Here's how the part is built. I have some questions about the finished solid (model axes, mm). A direction names the side the tool comes from. Give positions to 0.01 mm unless a question says otherwise; leave off trailing zeros. Loops run counter-clockwise (first coordinate to the right, second up) from the corner with the lowest first, then second, coordinate; pieces in that order, holes last. Notation, with made-up numbers: (-38.5, 71.5) - (18.5, 71.5) arc R16 cw to (18.5, 95.5) - close; hole circle Ø8 at (42, 88.25). An arc over 180 degrees is marked (long way). Use one line per item in the form item = value.
Autodesk Inventor part; units mm, degrees
ref_plane "YZ Plane" through (0, 0, 0) normal (1, 0, 0) x (0, 1, 0)
ref_plane "XZ Plane" through (0, 0, 0) normal (0, 1, 0) x (-1, 0, 0)
ref_plane "XY Plane" through (0, 0, 0) normal (0, 0, 1) x (1, 0, 0)
sketch "Sketch1" plane through (0, 0, 0) normal (0, 1, 0) x (-1, 0, 0)
  line L0 (27.5, 37.5) -> (-27.5, 37.5)
  line L1 (-27.5, 37.5) -> (-27.5, -37.5)
  line L2 (-27.5, -37.5) -> (27.5, -37.5)
  line L3 (27.5, -37.5) -> (27.5, 37.5)
  line L4 (27.5, 37.5) -> (-27.5, -37.5) construction
  line L5 (-27.5, 37.5) -> (27.5, -37.5) construction
  point P0 (0, 0)
  dimension "d0" = 75
  dimension "d1" = 55
extrude "Extrusion1" add sketch "Sketch1" along normal blind 18
sketch "Sketch2" plane through (0, 18, 0) normal (0, 1, 0) x (1, 0, 0)
  line L0 (-27.5, -37.5) -> (27.5, -37.5)
  line L1 (-8.5, -37.5) -> (-8.5, 37.5)
  line L2 (27.5, -37.5) -> (27.5, 37.5)
  line L3 (-8.5, 37.5) -> (27.5, 37.5)
  line L4 (-8.5, -37.5) -> (27.5, -37.5)
  dimension "d4" = 36
extrude "Extrusion2" add sketch "Sketch2" along normal blind 7
sketch "Sketch3" plane through (0, 18, 0) normal (0, 1, 0) x (1, 0, 0)
  line L0 (27.5, 37.5) -> (-27.5, 37.5)
  line L1 (-27.5, 37.5) -> (-27.5, -37.5)
  line L2 (-8.5, 37.5) -> (-8.5, -37.5)
  circle A0 centre (-18, 25.4407) radius 5.5
  circle A1 centre (-18, -24.214) radius 5.5
  point P0 (0, 0)
  dimension "d9" = 19
  dimension "d10" = 11
  dimension "d11" = 11
extrude "Extrusion3" cut sketch "Sketch3" against normal blind 7
sketch "Sketch4" plane through (-18, 11, -25.4407) normal (0, 1, 0) x (1, 0, 0)
  circle A0 centre (0, 0) radius 3.2
  circle A1 centre (0, -49.6547) radius 5.5
  circle A2 centre (0, -49.6547) radius 3.2
  point P0 (18, -25.4407)
  dimension "d14" = 6.4
  dimension "d15" = 6.4
extrude "Extrusion4" cut sketch "Sketch4" against normal blind 15 contours A0 | A2
sketch "Sketch5" plane through (0, 25, 0) normal (0, 1, 0) x (1, 0, 0)
  circle A0 centre (19.5, 0) radius 7.5
  circle A1 centre (4.5, 10.5) radius 7.5
  circle A2 centre (4.5, -10.5) radius 7.5
  line L0 (27.5, -37.5) -> (27.5, 37.5)
  point P0 (0, 0)
  dimension "d18" = 15
  dimension "d19" = 15
  dimension "d20" = 15
  dimension "d21" = 23
  dimension "d22" = 23
  dimension "d23" = 8
  dimension "d26" = 21
  dimension "d27" = 10.5
  dimension "d28" = 10.5
extrude "Extrusion5" cut sketch "Sketch5" against normal blind 10
sketch "Sketch6" plane through (4.5, 15, 10.5) normal (0, 1, 0) x (1, 0, 0)
  circle A0 centre (0, 0) radius 4.2
  circle A1 centre (0, 21) radius 7.5
  circle A2 centre (0, 21) radius 4.2
  circle A3 centre (15, 10.5) radius 7.5
  circle A4 centre (15, 10.5) radius 4.2
  point P0 (-4.5, 10.5)
  dimension "d29" = 8.4
  dimension "d30" = 8.4
  dimension "d31" = 8.4
extrude "Extrusion6" cut sketch "Sketch6" against normal blind 20 contours A0 | A2 | A4
properties part number "Feste Backe"
(1) For P1, Ø9, axis at x = -16, z = -24, coming from the +Y side; P2, Ø9.5, axis at x = 4.5, z = -10.5, coming from the +Y side; P3, Ø4, axis at x = -18, z = 24.214, coming from the +Y side; P4, Ø6.5, axis at x = -18, z = 24.214, coming from the +Y side, each with a flat end and sliding along its axis, tell me the tip position at first contact or that it passes through.
Geometry says:
P1 = 18
P2 = 15
P3 = through
P4 = 11
(2) If we section it at D-D (x = 20.5): List the corners of the cut face in (y, z) for me, plus the area to 3 significant figures.
Geometry says:
outline = (0, -37.5) - (25, -37.5) - (25, -7.43) - (15, -7.43) - (15, -4.08) - (0, -4.08) - close; (0, 4.08) - (15, 4.08) - (15, 7.43) - (25, 7.43) - (25, 37.5) - (0, 37.5) - close
area = 1,600 mm²
(3) If I drill on probe 1 along Z at (x, y) = (-18, 5.25); probe 2 along Z at (x, y) = (4.5, 8); probe 3 along X at (y, z) = (23.5, 0), over which ranges is the centre line in solid material (lowest first)?
Geometry says:
probe_1 = -37.5 to -28.64, -22.24 to 21.01, 27.41 to 37.5
probe_2 = -37.5 to -14.7, -6.3 to 6.3, 14.7 to 37.5
probe_3 = -8.5 to 12, 27 to 27.5
(4) For faces 5 (the flat face through (0, 0, 1)), 6 (the flat face through (8, 15, -7)), 7 (the flat face through (-18, 18, 1)), which set-ups out of +Z, -Z, +X, -X, +Y, -Y let a thin tool reach every point of the face, with its end or its side?
Geometry says:
face_5 = +Z, -Z, +X, -X, -Y
face_6 = +Y
face_7 = +Z, -Z, -X, +Y
(5) If we section it at A-A (x = -18): List the corners of the cut face in (y, z) for me, plus the area to 3 significant figures.
Geometry says:
outline = (0, -37.5) - (18, -37.5) - (18, -30.94) - (11, -30.94) - (11, -28.64) - (0, -28.64) - close; (0, -22.24) - (11, -22.24) - (11, -19.94) - (18, -19.94) - (18, 18.71) - (11, 18.71) - (11, 21.01) - (0, 21.01) - close; (0, 27.41) - (11, 27.41) - (11, 29.71) - (18, 29.71) - (18, 37.5) - (0, 37.5) - close
area = 1,060 mm²
(6) If we section it at B-B (y = 19.5): List the corners of the cut face in (x, z) for me, plus the area to 3 significant figures.
Geometry says:
outline = (-8.5, -37.5) - (27.5, -37.5) - (27.5, 37.5) - (-8.5, 37.5) - close; hole circle Ø15 at (4.5, -10.5); hole circle Ø15 at (4.5, 10.5); hole circle Ø15 at (19.5, 0)
area = 2,170 mm²
(7) Thinking about a two-plate mould opening in Z: for faces 1 (the cylindrical face through (3.953, 7.605, -14.664)), 2 (the flat face through (0, 12, -37.5)), 3 (the flat face through (27.5, 12, 1)), 4 (the cylindrical face through (2.87, 20.07, -3.18)), which applies, pulls with the +Z half, pulls with the -Z half, needs draft (parallel to the pull), parting line crosses it, or undercut?
Geometry says:
face_1 = undercut
face_2 = pulls with the -Z half
face_3 = needs draft
face_4 = undercut
(8) If we section it at C-C (z = 10.5): List the corners of the cut face in (x, y) for me, plus the area to 3 significant figures.
Geometry says:
outline = (-27.5, 0) - (0.3, 0) - (0.3, 15) - (-3, 15) - (-3, 25) - (-8.5, 25) - (-8.5, 18) - (-27.5, 18) - close; (8.7, 0) - (27.5, 0) - (27.5, 25) - (12, 25) - (12, 15) - (8.7, 15) - close
area = 966 mm²
